Autodesk Inventor part; units mm, degrees
ref_plane "YZ Plane" through (0, 0, 0) normal (1, 0, 0) x (0, 1, 0)
ref_plane "XZ Plane" through (0, 0, 0) normal (0, 1, 0) x (-1, 0, 0)
ref_plane "XY Plane" through (0, 0, 0) normal (0, 0, 1) x (1, 0, 0)
sketch "Sketch1" plane through (0, 0, 0) normal (0, 1, 0) x (-1, 0, 0)
  line L0 (0, 0) -> (-228.6, 0)
  line L1 (-228.6, 0) -> (-228.6, -76.2)
  line L2 (-228.6, -76.2) -> (-200.025, -76.2)
  line L3 (-200.025, -76.2) -> (-200.025, -44.45)
  line L4 (-200.025, -44.45) -> (-114.3, -44.45)
  line L5 (-114.3, -44.45) -> (-114.3, -50.8)
  line L6 (-114.3, -50.8) -> (-74.6125, -50.8)
  line L7 (-74.6125, -50.8) -> (-74.6125, -76.2)
  line L8 (-74.6125, -76.2) -> (0, -76.2)
  line L9 (0, -76.2) -> (0, 0)
  dimension "d0" = 228.6
  dimension "d2" = 76.2
  dimension "d3" = 28.575
  dimension "d4" = 31.75
  dimension "d5" = 85.725
  dimension "d6" = 6.35
  dimension "d7" = 39.6875
extrude "Extrusion1" add sketch "Sketch1" along normal blind 25.4
properties part number "StairTemplate"
Model file for the job. Use its own axes, mm. A direction names the side the tool comes from. Coordinates: 2 decimals unless noted, no trailing zeros. Write each loop counter-clockwise with the first axis right and the second up, starting at its lowest first coordinate (ties: lowest second). Pieces come first, ordered by that corner, then holes. Notation, with made-up numbers: (68, 16) - (84, 16) arc R4 cw to (84, 21) - close; hole circle Ø2 at (22.5, -12). An arc over 180 degrees is marked (long way). One line per item, written item: value. Start each with the question number.
1. Slice it at A-A (z = -60). Write the cut outline in (x, y) (1 decimal), plus the area to 3 significant figures.
2. Flat gauge pins, fed straight in: pin 1 (2 mm diameter, centred on x = 100.5, y = 15.5, fed in from -Z); pin 2 (12.5 mm diameter, centred on x = 152, y = 8, fed in from -Z). Where does each tip first touch, or does it go through?
3. Slice it at C-C (x = 171.5). Write the cut outline in (y, z), plus the area to 3 significant figures.
4. Probe line 1 (X direction, y = 23.75, z = -54) (1 decimal); line 2 (X direction, y = 15.25, z = -50) (3 decimals); line 3 (Z direction, x = 77, y = 7.75). List the from-to ranges inside material, lowest first. Write a range as from..to.
5. Mould opens along X. For faces 1 (the flat face through (113, 13, 0)), 2 (the flat face through (0, 13, -39)), 3 (the flat face through (158, 13, -44.45)) say: released by +X, released by -X, zero draft, split by the parting line, or undercut.
6. Tool access for faces 4 (the flat face through (38, 13, -76.2)), 5 (the flat face through (200.025, 13, -61)): list every direction of +Z, -Z, +X, -X, +Y, -Y with a clear straight run to the whole face (end or side of a thin tool).
7. Slice it at D-D (x = 95). Write the cut outline in (y, z).
Answers below:
1. outline: (0, 0) - (74.6, 0) - (74.6, 25.4) - (0, 25.4) - close; (200, 0) - (228.6, 0) - (228.6, 25.4) - (200, 25.4) - close
1. area: 2,620 mm^2
2. pin 1: stops at z = -50.8
2. pin 2: stops at z = -44.45
3. outline: (0, -44.45) - (25.4, -44.45) - (25.4, 0) - (0, 0) - close
3. area: 1,130 mm^2
4. line 1: x = 0..74.6, 200..228.6
4. line 2: x = 0..114.3, 200.025..228.6
4. line 3: z = -50.8..0
5. face 1: zero draft
5. face 2: released by -X
5. face 3: undercut
6. face 4: -Z, +X, -X, +Y, -Y
6. face 5: -Z, +Y, -Y
7. outline: (0, -50.8) - (25.4, -50.8) - (25.4, 0) - (0, 0) - close
